from build123d import *

# Parameters (mm, degrees)
SKETCH1_R           = 51.054
BOSS_EXTRUDE1_DEPTH = 25.4
SKETCH2_R           = 4.365625
CUT_EXTRUDE1_DEPTH  = 31.75
CIRPATTERN1_COUNT   = 8
SKETCH3_R           = 48.26
BOSS_EXTRUDE2_DEPTH = 2.54


with BuildPart() as part:
    # Sketch1 → Boss-Extrude1 (new body)
    with BuildSketch(Plane(origin=(0, 0, 0), x_dir=(1, 0, 0), z_dir=(0, 1, 0))):
        Polygon((63.5, 26.302561211), (26.302561211, 63.5), (-26.302561211, 63.5), (-63.5, 26.302561211), (-63.5, -26.302561211), (-26.302561211, -63.5), (26.302561211, -63.5), (63.5, -26.302561211), align=None)
        with Locations(Location((0, 0, 0), (0, 0, 270))):
            Circle(SKETCH1_R, mode=Mode.SUBTRACT)
    extrude(amount=BOSS_EXTRUDE1_DEPTH)

    # Sketch2 → Cut-Extrude1 (cut)
    with BuildSketch(Plane(origin=(63.5, 0, 0), x_dir=(0, 0, -1), z_dir=(1, 0, 0))):
        with Locations((0, 12.7)):
            Circle(SKETCH2_R)
    cut_extrude1 = extrude(amount=-CUT_EXTRUDE1_DEPTH, mode=Mode.SUBTRACT)

    # CirPattern1: Cut-Extrude1 ×8 about axis
    cirpattern1_axis = Axis((0, 25.4, 0), (0, -1, 0))
    for i in range(1, CIRPATTERN1_COUNT):
        add(cut_extrude1.rotate(cirpattern1_axis, i * 360 / CIRPATTERN1_COUNT), mode=Mode.SUBTRACT)

    # Sketch3 → Boss-Extrude2 (add)
    with BuildSketch(Plane.XZ):
        Polygon((26.302561211, 63.5), (-26.302561211, 63.5), (-63.5, 26.302561211), (-63.5, -26.302561211), (-26.302561211, -63.5), (26.302561211, -63.5), (63.5, -26.302561211), (63.5, 26.302561211), align=None)
        with Locations(Location((0, 0, 0), (0, 0, 270))):
            Circle(SKETCH3_R, mode=Mode.SUBTRACT)
    extrude(amount=BOSS_EXTRUDE2_DEPTH)


solid = part.part
Check sheet for the modelled part. Datum: model origin and axes. Units: mm. A direction names the side the tool comes from. Give positions to 0.01 mm unless a question says otherwise; leave off trailing zeros. Write each loop counter-clockwise with the first axis right and the second up, starting at its lowest first coordinate (ties: lowest second). Pieces come first, ordered by that corner, then holes. Notation, with made-up numbers: (-34.5, -26) -> (12.5, -26) arc R19 cw to (12.5, -13) -> close; hole circle Ø6 at (32, 69). An arc over 180 degrees is marked (long way). Use one line per item in the form item = value. Start each with the question number.
1. Section check C-C (y = 3). Record the cut outline in (x, z), and give its area (3 significant figures).
2. Thickness scan on line 1 along Z through (x, y) = (0, 20); line 2 along Y through (x, z) = (0, 58); line 3 along X through (y, z) = (-0.55, 0). Record the ranges inside material, lowest first. Write a range as from..to.
3. Access from +Z, -Z, +X, -X, +Y, -Y to the whole of each face (thin tool, end or side, straight path). Record for faces 5 (the flat face through (38, 0, 30)), 6 (the flat face through (-48.8, 11.6, 41)).
4. Section check B-B (x = 0). Record the cut outline in (y, z).
5. Go/stop test with flat-tipped pins: P1, Ø5, axis at x = 38.5, z = 26, coming from the +Y side; P2, Ø2, axis at y = 8, z = -48.5, coming from the -X side; P3, Ø10, axis at y = 10, z = -46, coming from the -X side. Record where each tip stops, or that it passes through.
6. Section check A-A (z = 0). Record the cut outline in (x, y).
7. Section check D-D (z = 31). Record the cut outline in (x, y).
8. Mould release check, pull along X, two halves, no side actions. Record for faces 1 (the flat face through (-41, 11.6, -48.8)), 2 (the flat face through (63.5, 12, 5)), 3 (the flat face through (-5, 25.4, 51)), 4 (the cylindrical face through (-19.554, 12.522, 47.161)): pulls with the +X half, pulls with the -X half, needs draft (parallel to the pull), parting line crosses it, or undercut.
Conclusion:
q1.outline = (-63.5, -26.3) -> (-26.3, -63.5) -> (26.3, -63.5) -> (63.5, -26.3) -> (63.5, 26.3) -> (26.3, 63.5) -> (-26.3, 63.5) -> (-63.5, 26.3) -> close; hole circle Ø102.11 at (0, 0)
q1.area = 5,170 mm²
q2.line_1 = -63.5..-51.05, 51.05..63.5
q2.line_2 = -2.54..8.33, 17.07..25.4
q2.line_3 = -63.5..-48.26, 48.26..63.5
q3.face_5 = +Y
q3.face_6 = +Z, -X, +Y, -Y
q4.outline = (-2.54, -63.5) -> (8.33, -63.5) -> (8.33, -51.05) -> (0, -51.05) -> (0, -48.26) -> (-2.54, -48.26) -> close; (-2.54, 48.26) -> (0, 48.26) -> (0, 51.05) -> (8.33, 51.05) -> (8.33, 63.5) -> (-2.54, 63.5) -> close; (17.07, -63.5) -> (25.4, -63.5) -> (25.4, -51.05) -> (17.07, -51.05) -> close; (17.07, 51.05) -> (25.4, 51.05) -> (25.4, 63.5) -> (17.07, 63.5) -> close
q5.P1 = 0
q5.P2 = -42.3
q5.P3 = -48.8
q6.outline = (-63.5, -2.54) -> (-48.26, -2.54) -> (-48.26, 0) -> (-51.05, 0) -> (-51.05, 8.33) -> (-63.5, 8.33) -> close; (-63.5, 17.07) -> (-51.05, 17.07) -> (-51.05, 25.4) -> (-63.5, 25.4) -> close; (48.26, -2.54) -> (63.5, -2.54) -> (63.5, 8.33) -> (51.05, 8.33) -> (51.05, 0) -> (48.26, 0) -> close; (51.05, 17.07) -> (63.5, 17.07) -> (63.5, 25.4) -> (51.05, 25.4) -> close
q7.outline = (-58.8, -2.54) -> (-36.99, -2.54) -> (-36.99, 0) -> (-40.56, 0) -> (-40.56, 25.4) -> (-58.8, 25.4) -> close; (36.99, -2.54) -> (58.8, -2.54) -> (58.8, 25.4) -> (40.56, 25.4) -> (40.56, 0) -> (36.99, 0) -> close
q8.face_1 = pulls with the -X half
q8.face_2 = pulls with the +X half
q8.face_3 = needs draft
q8.face_4 = undercut
